Geometry: final body of the model. Coordinates: model frame, mm. Face numbers are marked on the shaded views. A direction names the side the tool comes from. Round coordinates to 2 decimals unless told otherwise and drop trailing zeros. Order: outer loops, then holes, each group sorted by start corner. A loop starts at its lowest first (then second) coordinate and runs counter-clockwise, first axis right, second up. Notation, with made-up numbers: (0, 56) -> (55, 56) arc R17 ccw to (55, 67) -> close; hole circle Ø5 at (55, 24). An arc over 180 degrees is marked (long way). Put each result on its own line as item: value.
Autodesk Inventor part; units mm, degrees
ref_plane "Work Plane4" through (-67.5, 9.7, -88) normal (-1, 0, 0) x (0, 0, 1)
ref_plane "Work Plane5" through (-62.5, 9.7, -88) normal (1, 0, 0) x (0, 0, -1)
ref_plane "Work Plane3" through (0, 22.5, 0) normal (0, 1, 0) x (1, 0, 0)
sketch "Sketch1" plane through (0, 0, 0) normal (0, 1, 0) x (-1, 0, 0)
  line L0 (-67.5, 75) -> (67.5, 75)
  line L1 (67.5, 75) -> (67.5, -75)
  line L2 (67.5, -75) -> (-67.5, -75)
  line L3 (-67.5, -75) -> (-67.5, 75)
  line L4 (-67.5, 75) -> (67.5, -75) construction
  line L5 (67.5, 75) -> (-67.5, -75) construction
  point P0 (0, 0)
  dimension "d0" = 135
  dimension "d1" = 150
extrude "Extrusion1" add sketch "Sketch1" along normal blind 8
sketch "Sketch3" plane through (0, 8, 0) normal (0, 1, 0) x (1, 0, 0)
  line L0 (-67.5, -75) -> (67.5, -75)
  line L1 (67.5, -75) -> (67.5, 75)
  line L2 (67.5, 75) -> (-67.5, 75)
  line L3 (-67.5, 75) -> (-67.5, -75)
  line L4 (62.5, 75) -> (62.5, -70)
  line L5 (-67.5, -75) -> (67.5, -75)
  line L6 (67.5, -75) -> (67.5, 75)
  line L7 (0, 0) -> (0, -83) construction
  line L8 (-62.5, 75) -> (-62.5, -70)
  line L9 (62.5, -70) -> (-62.5, -70)
  dimension "d4" = 5
  dimension "d5" = 5
extrude "Extrusion2" add sketch "Sketch3" along normal blind 38.7 contours L3 L2 L8 L9 L4 L1 L0
sketch "Sketch4" plane through (67.5, 0, -75) normal (0, 0, -1) x (-1, 0, 0)
  line L0 (135, 0) -> (0, 0)
  line L1 (135, 0) -> (135, 46.7)
  line L2 (130, 46.7) -> (135, 46.7)
  line L3 (130, 8) -> (130, 46.7)
  line L4 (5, 8) -> (130, 8)
  line L5 (5, 8) -> (5, 46.7)
  line L6 (0, 46.7) -> (5, 46.7)
  line L7 (0, 0) -> (0, 46.7)
  line L8 (130, 8) -> (5, 8)
  line L9 (5, 8) -> (5, 0)
  line L10 (130, 8) -> (130, 0)
  line L11 (0, 0) -> (135, 0)
  line L12 (0, 0) -> (0, 46.7)
  line L13 (5, 3) -> (130, 3)
  line L14 (5, 8) -> (130, 8)
  line L15 (5, 6) -> (130, 6)
  line L16 (5, 8) -> (0, 8)
  line L17 (135, 0) -> (0, 0)
  point P0 (67.5, 0)
  dimension "d8" = 3
  dimension "d9" = 3
extrude "Extrusion3" add sketch "Sketch4" along normal blind 20 contours L0 L10 L3 L2 L1 | L0 L9 L13 L10 | L15 L9 L4 L10 | L7 L6 L5 L16
sketch "Sketch6" plane through (67.5, 0, 75) normal (1, 0, 0) x (0, 0, -1)
  line L0 (150, 0) -> (150, 8)
  line L1 (0, 0) -> (0, 46.7)
  line L2 (150, 8) -> (170, 8)
  line L3 (0, 46.7) -> (170, 46.7)
  line L4 (170, 46.7) -> (170, 8)
  line L5 (170, 21) -> (153, 21)
  line L6 (153, 21) -> (153, 33)
  line L7 (153, 33) -> (170, 33)
  line L8 (170, 33) -> (170, 21)
  point P0 (75, 0)
  dimension "d92" = 13
  dimension "d93" = 17
  dimension "d94" = 12
fillet "Fillet1" radius 2 11 edges at (67.5, 0, 0) (67.5, 46.7, -10) (67.5, 23.35, 75) (0, 46.7, 75) (0, 0, 75) (-67.5, 46.7, -10) (-67.5, 23.35, 75) (-67.5, 0, -10) (62.5, 46.7, -12.5) (-62.5, 46.7, -12.5) (0, 46.7, 70)
ref_plane "Work Plane4" through (-67.5, 9.7, -88) normal (-1, 0, 0) x (0, 0, 1)
sketch "Sketch15" plane through (62.5, 6, -75) normal (1, 0, 0) x (0, 0, -1)
  line L0 (0, 0) -> (0, 2)
  line L1 (0, 0) -> (20, 0)
  line L2 (20, 2) -> (20, 0)
  line L3 (0, 2) -> (20, 2)
  point P0 (-75, -6)
extrude "Extrusion8" add sketch "Sketch15" along normal blind 2.5
sketch "Sketch16" plane through (0, 8, 0) normal (0, 1, 0) x (1, 0, 0)
  line L0 (-62.5, -35) -> (-46.5, -35)
  line L1 (-46.5, -35) -> (-46.5, 5)
  line L2 (-46.5, 5) -> (-62.5, 5)
  line L3 (-62.5, 5) -> (-62.5, -35)
  line L4 (62.5, -70) -> (-62.5, -70)
  line L5 (-62.5, -70) -> (-62.5, 95)
  line L6 (46.5, -70) -> (62.5, -70)
  line L7 (62.5, -70) -> (62.5, -30)
  line L8 (62.5, -30) -> (46.5, -30)
  line L9 (46.5, -30) -> (46.5, -70)
  line L10 (62.5, 95) -> (62.5, -70)
  point P0 (0, 0)
  dimension "d39" = 35
  dimension "d40" = 0
  dimension "d41" = 16
  dimension "d42" = 40
  dimension "d43" = 0
  dimension "d44" = 0
  dimension "d45" = 40
  dimension "d46" = 16
extrude "Extrusion9" add sketch "Sketch16" along normal blind 16
fillet "Fillet4" radius 1 8 edges at (46.5, 24, 50) (54.5, 24, 30) (46.5, 16, 30) (-46.5, 24, 15) (-46.5, 16, -5) (-54.5, 24, 35) (-54.5, 24, -5) (-46.5, 16, 35)
sketch "Sketch17" plane through (0, 24, 0) normal (0, 1, 0) x (1, 0, 0)
  circle A0 centre (-56.5, -25) radius 2.25
  line L0 (-62.5, -34) -> (-62.5, 4)
  line L1 (-47.5, -34) -> (-62.5, -34)
  circle A1 centre (54.5, -57.5) radius 2.25
  line L2 (47.5, -70) -> (47.5, -31)
  line L3 (47.5, -31) -> (62.5, -31)
  line L4 (62.5, -70) -> (50.5, -70)
  point P0 (0, 0)
  dimension "d50" = 4.5
  dimension "d51" = 6
  dimension "d52" = 9
  dimension "d53" = 4.5
  dimension "d54" = 7
  dimension "d90" = 12.5
extrude "Extrusion10" cut sketch "Sketch17" against normal blind 12
ref_plane "Work Plane5" through (-62.5, 9.7, -88) normal (1, 0, 0) x (0, 0, -1)
sketch "Sketch18" plane through (-62.5, 9.7, -88) normal (1, 0, 0) x (0, 0, -1)
  circle A0 centre (-68, 19) radius 2.25
  circle A1 centre (-37.2, 19) radius 2.25
  line L0 (0, 8.1) -> (0, 14.1)
  line L1 (-37.2, 19) -> (-68, 19)
  line L2 (7, 37) -> (-160, 37)
  line L3 (-158, -1.7) -> (-158, 35)
  point P0 (-88, -9.7)
  dimension "d60" = 4.5
  dimension "d61" = 4.5
  dimension "d62" = 30.8
  dimension "d67" = 90
  dimension "d91" = 18
extrude "Extrusion11" cut sketch "Sketch18" against normal through all
ref_plane "Work Plane3" through (0, 22.5, 0) normal (0, 1, 0) x (1, 0, 0)
sketch "Sketch21" plane through (0, 22.5, 0) normal (0, 1, 0) x (1, 0, 0)
  circle A0 centre (54.5, -57.5) radius 2.25
  line L0 (50.75, -55.3349) -> (54.5, -53.1699)
  line L1 (54.5, -53.1699) -> (58.25, -55.3349)
  line L2 (58.25, -55.3349) -> (58.25, -59.6651)
  line L3 (58.25, -59.6651) -> (54.5, -61.8301)
  line L4 (54.5, -61.8301) -> (50.75, -59.6651)
  line L5 (50.75, -59.6651) -> (50.75, -55.3349)
  line L6 (-62.5, -35) -> (-62.5, -70)
  line L7 (46.5, -70) -> (46.5, -31)
  circle A1 centre (-56.5, -25) radius 2.25
  line L8 (-52.75, -27.1651) -> (-56.5, -29.3301)
  line L9 (-56.5, -29.3301) -> (-60.25, -27.1651)
  line L10 (-60.25, -27.1651) -> (-60.25, -22.8349)
  line L11 (-60.25, -22.8349) -> (-56.5, -20.6699)
  line L12 (-56.5, -20.6699) -> (-52.75, -22.8349)
  line L13 (-52.75, -22.8349) -> (-52.75, -27.1651)
  point P0 (0, 0)
  dimension "d78" = 7.5
  dimension "d79" = 7.5
extrude "Extrusion13" cut sketch "Sketch21" against normal blind 3.15
extrude "Extrusion14" cut sketch "Sketch6" against normal through all
properties part number "Case_metà1"
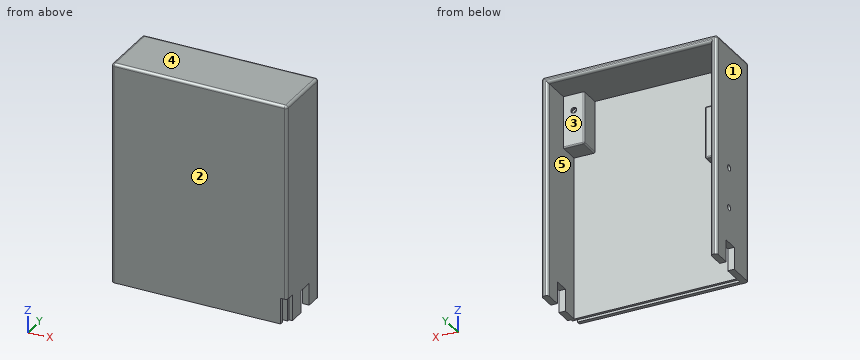
1. Cut plane C-C on x = -15.5. Return loops of the section in (y, z), and give its area (3 significant figures).
Ans:
outline: (0, -95) -> (3, -95) -> (3, -75) -> (6, -75) -> (6, -95) -> (8, -95) -> (8, 70) -> (44.7, 70) arc R2 ccw to (46.7, 72) -> (46.7, 73) arc R2 ccw to (44.7, 75) -> (2, 75) arc R2 ccw to (0, 73) -> close
area: 1,490 mm²
2. Cut plane A-A on y = 28.7. Return loops of the section in (x, z), and give its area (3 significant figures).
Ans:
outline: (-67.5, -78) -> (-62.5, -78) -> (-62.5, -53.05) -> (-67.5, -53.05) -> close; (-67.5, -48.55) -> (-62.5, -48.55) -> (-62.5, -22.25) -> (-67.5, -22.25) -> close; (-67.5, -17.75) -> (-62.5, -17.75) -> (-62.5, 70) -> (62.5, 70) -> (62.5, -78) -> (67.5, -78) -> (67.5, 73) arc R2 ccw to (65.5, 75) -> (-65.5, 75) arc R2 ccw to (-67.5, 73) -> close
area: 2,110 mm²
3. Cut plane B-B on z = -50.8. Return loops of the section in (x, y), and give its area (3 significant figures).
Ans:
outline: (-67.5, 2) arc R2 ccw to (-65.5, 0) -> (65.5, 0) arc R2 ccw to (67.5, 2) -> (67.5, 44.7) arc R2 ccw to (65.5, 46.7) -> (64.5, 46.7) arc R2 ccw to (62.5, 44.7) -> (62.5, 8) -> (-62.5, 8) -> (-62.5, 26.45) -> (-67.5, 26.45) -> close; (-67.5, 30.95) -> (-62.5, 30.95) -> (-62.5, 44.7) arc R2 ccw to (-64.5, 46.7) -> (-65.5, 46.7) arc R2 ccw to (-67.5, 44.7) -> close
area: 1,440 mm²
4. Contact query for flat-ended pins moving along their axis: P1, Ø3.5, axis at x = -55.5, z = 25, coming from the +Y side; P2, Ø0.6, axis at y = 7, z = -87.5, coming from the +X side; P3, Ø1.5, axis at x = 17, z = -41.5, coming from the +Y side. Output: stop coordinate, or through.
Ans:
P1: y = 24
P2: x = 65
P3: y = 8
5. Draft query along X for the marked faces 1, 2 and 3. Return one class per face: +X half, -X half, draft (parallel to the pull), parting line (faces both ways), or undercut.
Ans:
face 1: -X half
face 2: draft
face 3: undercut
6. Set-up query: the marked faces 4 and 5. Return all of +Z, -Z, +X, -X, +Y, -Y with unobstructed straight access to the full face (end or side cutting, diameter ignored); none if empty.
Ans:
face 4: +Z, +X, -X, +Y, -Y
face 5: -Z, +Y
7. Cut plane D-D on y = 14. Return loops of the section in (x, z), and give its area (3 significant figures).
Ans:
outline: (-67.5, -95) -> (-62.5, -95) -> (-62.5, -5) -> (-47.5, -5) arc R1 ccw to (-46.5, -4) -> (-46.5, 34) arc R1 ccw to (-47.5, 35) -> (-62.5, 35) -> (-62.5, 70) -> (46.5, 70) -> (46.5, 31) arc R1 ccw to (47.5, 30) -> (62.5, 30) -> (62.5, -95) -> (67.5, -95) -> (67.5, 73) arc R2 ccw to (65.5, 75) -> (-65.5, 75) arc R2 ccw to (-67.5, 73) -> close; hole circle Ø4.5 at (-56.5, 25); hole circle Ø4.5 at (54.5, 57.5)
area: 3,570 mm²
8. Material intervals for probe 1 along Z at (x, y) = (-56.5, 15.5); probe 2 along X at (y, z) = (17.5, 25); probe 3 along X at (y, z) = (23.1, 57.5), sorted ascending.
Ans:
probe 1: -5 to 22.75, 27.25 to 35, 70 to 75
probe 2: -67.5 to -58.75, -54.25 to -46.5, 62.5 to 67.5
probe 3: -67.5 to -62.5, 46.51 to 52.25, 56.75 to 67.5
